Could you check a few things on this model? Use its own coordinates, in mm. Give positions to 0.01 mm unless a question says otherwise; leave off trailing zeros.
1. I need wall thicknesses on line 1 along Y through (x, z) = (2296.5, 14); line 2 along Y through (x, z) = (2312.25, 122.5); line 3 along X through (y, z) = (1183, 25.5). Which ranges of each line are inside material? Lowest first, please.
2. For P1, Ø2.5, axis at x = 2296.61, y = 1180.19, coming from the +Z side; P2, Ø1, axis at x = 2301.5, z = 70, coming from the -Y side; P3, Ø1.5, axis at y = 1189, z = 66, coming from the -X side, each with a flat end and sliding along its axis, tell me the tip position at first contact or that it passes through.
3. Imagine slicing it at A-A (z = 76). Count the separate pieces of the cut face and the enclosed holes in it, plus the area to 3 significant figures.
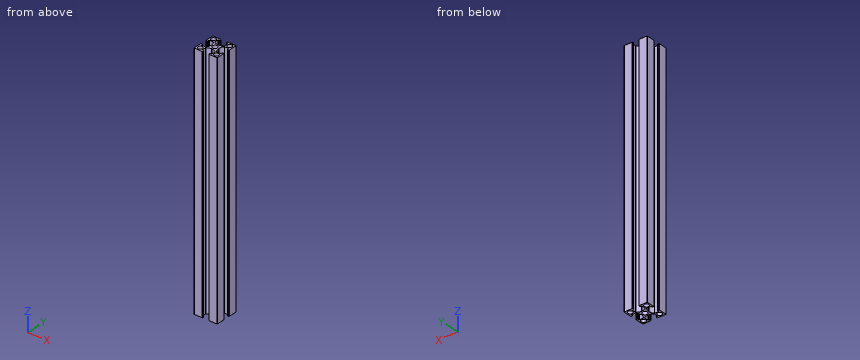
```python
from build123d import *

# Parameters (mm, degrees)
MODEL_R         = 2.15
MODEL_R_2       = 2
EXTRUDE_1_DEPTH = 208.5


with BuildPart() as part:
    # Model → 보스-돌출1 (new body)
    with BuildSketch(Plane.XY):
        with BuildLine():
            Line((2307.763927197, 1192.134297913), (2307.763927197, 1195.391548465))
            ThreePointArc((2307.763927197, 1195.391548465), (2307.676059232, 1195.603680499), (2307.463927197, 1195.691548465))
            Line((2307.463927197, 1195.691548465), (2306.563927197, 1195.691548465))
            ThreePointArc((2306.563927197, 1195.691548465), (2306.351795163, 1195.779416431), (2306.263927197, 1195.991548465))
            Line((2306.263927197, 1195.991548465), (2306.263927197, 1196.891548465))
            ThreePointArc((2306.263927197, 1196.891548465), (2306.351795163, 1197.103680499), (2306.563927197, 1197.191548465))
            Line((2306.563927197, 1197.191548465), (2313.313927197, 1197.191548465))
            ThreePointArc((2313.313927197, 1197.191548465), (2313.526059232, 1197.103680499), (2313.613927197, 1196.891548465))
            Line((2313.613927197, 1196.891548465), (2313.613927197, 1190.141548465))
            ThreePointArc((2313.613927197, 1190.141548465), (2313.526059232, 1189.929416431), (2313.313927197, 1189.841548465))
            Line((2313.313927197, 1189.841548465), (2312.413927197, 1189.841548465))
            ThreePointArc((2312.413927197, 1189.841548465), (2312.201795163, 1189.929416431), (2312.113927197, 1190.141548465))
            Line((2312.113927197, 1190.141548465), (2312.113927197, 1191.041548465))
            ThreePointArc((2312.113927197, 1191.041548465), (2312.026059232, 1191.253680499), (2311.813927197, 1191.341548465))
            Line((2311.813927197, 1191.341548465), (2308.556676645, 1191.341548465))
            ThreePointArc((2308.556676645, 1191.341548465), (2308.426234796, 1191.311705686), (2308.321744595, 1191.228114625))
            ThreePointArc((2308.321744595, 1191.228114625), (2307.328306374, 1189.47356999), (2306.921204563, 1187.498825831))
            Line((2306.921204563, 1187.498825831), (2306.613927197, 1187.191548465))
            Line((2306.613927197, 1187.191548465), (2306.921204563, 1186.884271099))
            ThreePointArc((2306.921204563, 1186.884271099), (2307.328306374, 1184.90952694), (2308.321744595, 1183.154982305))
            ThreePointArc((2308.321744595, 1183.154982305), (2308.426234796, 1183.071391244), (2308.556676645, 1183.041548465))
            Line((2308.556676645, 1183.041548465), (2311.813927197, 1183.041548465))
            ThreePointArc((2311.813927197, 1183.041548465), (2312.026059232, 1183.129416431), (2312.113927197, 1183.341548465))
            Line((2312.113927197, 1183.341548465), (2312.113927197, 1184.241548465))
            ThreePointArc((2312.113927197, 1184.241548465), (2312.201795163, 1184.453680499), (2312.413927197, 1184.541548465))
            Line((2312.413927197, 1184.541548465), (2313.313927197, 1184.541548465))
            ThreePointArc((2313.313927197, 1184.541548465), (2313.526059232, 1184.453680499), (2313.613927197, 1184.241548465))
            Line((2313.613927197, 1184.241548465), (2313.613927197, 1177.491548465))
            ThreePointArc((2313.613927197, 1177.491548465), (2313.526059232, 1177.279416431), (2313.313927197, 1177.191548465))
            Line((2313.313927197, 1177.191548465), (2306.563927197, 1177.191548465))
            ThreePointArc((2306.563927197, 1177.191548465), (2306.351795163, 1177.279416431), (2306.263927197, 1177.491548465))
            Line((2306.263927197, 1177.491548465), (2306.263927197, 1178.391548465))
            ThreePointArc((2306.263927197, 1178.391548465), (2306.351795163, 1178.603680499), (2306.563927197, 1178.691548465))
            Line((2306.563927197, 1178.691548465), (2307.463927197, 1178.691548465))
            ThreePointArc((2307.463927197, 1178.691548465), (2307.676059232, 1178.779416431), (2307.763927197, 1178.991548465))
            Line((2307.763927197, 1178.991548465), (2307.763927197, 1182.248799017))
            ThreePointArc((2307.763927197, 1182.248799017), (2307.734084418, 1182.379240866), (2307.650493357, 1182.483731067))
            ThreePointArc((2307.650493357, 1182.483731067), (2305.895948722, 1183.477169289), (2303.921204563, 1183.884271099))
            Line((2303.921204563, 1183.884271099), (2303.613927197, 1184.191548465))
            Line((2303.613927197, 1184.191548465), (2303.306649831, 1183.884271099))
            ThreePointArc((2303.306649831, 1183.884271099), (2301.331905673, 1183.477169289), (2299.577361038, 1182.483731067))
            ThreePointArc((2299.577361038, 1182.483731067), (2299.493769977, 1182.379240866), (2299.463927197, 1182.248799017))
            Line((2299.463927197, 1182.248799017), (2299.463927197, 1178.991548465))
            ThreePointArc((2299.463927197, 1178.991548465), (2299.551795163, 1178.779416431), (2299.763927197, 1178.691548465))
            Line((2299.763927197, 1178.691548465), (2300.663927197, 1178.691548465))
            ThreePointArc((2300.663927197, 1178.691548465), (2300.876059232, 1178.603680499), (2300.963927197, 1178.391548465))
            Line((2300.963927197, 1178.391548465), (2300.963927197, 1177.491548465))
            ThreePointArc((2300.963927197, 1177.491548465), (2300.876059232, 1177.279416431), (2300.663927197, 1177.191548465))
            Line((2300.663927197, 1177.191548465), (2293.913927197, 1177.191548465))
            ThreePointArc((2293.913927197, 1177.191548465), (2293.701795163, 1177.279416431), (2293.613927197, 1177.491548465))
            Line((2293.613927197, 1177.491548465), (2293.613927197, 1184.241548465))
            ThreePointArc((2293.613927197, 1184.241548465), (2293.701795163, 1184.453680499), (2293.913927197, 1184.541548465))
            Line((2293.913927197, 1184.541548465), (2294.813927197, 1184.541548465))
            ThreePointArc((2294.813927197, 1184.541548465), (2295.026059232, 1184.453680499), (2295.113927197, 1184.241548465))
            Line((2295.113927197, 1184.241548465), (2295.113927197, 1183.341548465))
            ThreePointArc((2295.113927197, 1183.341548465), (2295.201795163, 1183.129416431), (2295.413927197, 1183.041548465))
            Line((2295.413927197, 1183.041548465), (2298.671177749, 1183.041548465))
            ThreePointArc((2298.671177749, 1183.041548465), (2298.801619599, 1183.071391244), (2298.906109799, 1183.154982305))
            ThreePointArc((2298.906109799, 1183.154982305), (2299.899548021, 1184.90952694), (2300.306649831, 1186.884271099))
            Line((2300.306649831, 1186.884271099), (2300.613927197, 1187.191548465))
            Line((2300.613927197, 1187.191548465), (2300.306649831, 1187.498825831))
            ThreePointArc((2300.306649831, 1187.498825831), (2299.899548021, 1189.47356999), (2298.906109799, 1191.228114625))
            ThreePointArc((2298.906109799, 1191.228114625), (2298.801619599, 1191.311705686), (2298.671177749, 1191.341548465))
            Line((2298.671177749, 1191.341548465), (2295.413927197, 1191.341548465))
            ThreePointArc((2295.413927197, 1191.341548465), (2295.201795163, 1191.253680499), (2295.113927197, 1191.041548465))
            Line((2295.113927197, 1191.041548465), (2295.113927197, 1190.141548465))
            ThreePointArc((2295.113927197, 1190.141548465), (2295.026059232, 1189.929416431), (2294.813927197, 1189.841548465))
            Line((2294.813927197, 1189.841548465), (2293.913927197, 1189.841548465))
            ThreePointArc((2293.913927197, 1189.841548465), (2293.701795163, 1189.929416431), (2293.613927197, 1190.141548465))
            Line((2293.613927197, 1190.141548465), (2293.613927197, 1196.891548465))
            ThreePointArc((2293.613927197, 1196.891548465), (2293.701795163, 1197.103680499), (2293.913927197, 1197.191548465))
            Line((2293.913927197, 1197.191548465), (2300.663927197, 1197.191548465))
            ThreePointArc((2300.663927197, 1197.191548465), (2300.876059232, 1197.103680499), (2300.963927197, 1196.891548465))
            Line((2300.963927197, 1196.891548465), (2300.963927197, 1195.991548465))
            ThreePointArc((2300.963927197, 1195.991548465), (2300.876059232, 1195.779416431), (2300.663927197, 1195.691548465))
            Line((2300.663927197, 1195.691548465), (2299.763927197, 1195.691548465))
            ThreePointArc((2299.763927197, 1195.691548465), (2299.551795163, 1195.603680499), (2299.463927197, 1195.391548465))
            Line((2299.463927197, 1195.391548465), (2299.463927197, 1192.134297913))
            ThreePointArc((2299.463927197, 1192.134297913), (2299.493769977, 1192.003856063), (2299.577361038, 1191.899365863))
            ThreePointArc((2299.577361038, 1191.899365863), (2301.331905673, 1190.905927641), (2303.306649831, 1190.498825831))
            Line((2303.306649831, 1190.498825831), (2303.613927197, 1190.191548465))
            Line((2303.613927197, 1190.191548465), (2303.921204563, 1190.498825831))
            ThreePointArc((2303.921204563, 1190.498825831), (2305.895948722, 1190.905927641), (2307.650493357, 1191.899365863))
            ThreePointArc((2307.650493357, 1191.899365863), (2307.734084418, 1192.003856063), (2307.763927197, 1192.134297913))
        make_face()
        with Locations((2303.613927197, 1187.191548465)):
            Circle(MODEL_R, mode=Mode.SUBTRACT)
        with Locations((2296.613927197, 1194.191548465)):
            Circle(MODEL_R_2, mode=Mode.SUBTRACT)
        with Locations((2296.613927197, 1180.191548465)):
            Circle(MODEL_R_2, mode=Mode.SUBTRACT)
        with Locations((2310.613927197, 1194.191548465)):
            Circle(MODEL_R_2, mode=Mode.SUBTRACT)
        with Locations((2310.613927197, 1180.191548465)):
            Circle(MODEL_R_2, mode=Mode.SUBTRACT)
    extrude(amount=EXTRUDE_1_DEPTH)


solid = part.part
```
Derived:
1. line 1: y = 1177.19 to 1178.19, 1182.19 to 1183.04, 1191.34 to 1192.19, 1196.19 to 1197.19
1. line 2: y = 1177.19 to 1179.04, 1181.34 to 1184.49, 1189.89 to 1193.04, 1195.34 to 1197.19
1. line 3: x = 2293.61 to 2300.33, 2306.9 to 2313.61
2. P1: passes through
2. P2: stops at y = 1183.34
2. P3: stops at x = 2299.79
3. separate pieces: 1
3. enclosed holes: 5
3. area: 146 mm2
